Verification items for the finished model (mm, model axes). Face numbers are marked on the shaded views. A direction names the side the tool comes from. Coordinates: 2 decimals unless noted, no trailing zeros. Write each loop counter-clockwise with the first axis right and the second up, starting at its lowest first coordinate (ties: lowest second). Pieces come first, ordered by that corner, then holes. Notation, with made-up numbers: (6, 47) - (51, 47) arc R11 ccw to (51, 56) - close; hole circle Ø11 at (22, 68.5). An arc over 180 degrees is marked (long way). Use CSV: the item, a comma, the result in double quotes. Start each with the question number.
```python
from build123d import *

# Parameters (mm, degrees)
F0_R     = 9.5
F1_DEPTH = 20
F2_DEPTH = 15


with BuildPart() as f1:
    # F0 (on Top) → F1 (new body)
    with BuildSketch(Plane.XY):
        with BuildLine():
            ThreePointArc((11, 0), (2.57123, 10.695269), (-9.797959, 5))
            ThreePointArc((-9.797959, 5), (-11, 0), (-9.797959, -5))
            ThreePointArc((-9.797959, -5), (2.57123, -10.695269), (11, 0))
        make_face()
        Circle(F0_R, mode=Mode.SUBTRACT)
    extrude(amount=F1_DEPTH)

    # F0 (on Top) → F2 (join)
    with BuildSketch(Plane.XY):
        with BuildLine():
            Line((-9.797959, 5), (-24.797959, 5))
            Line((-24.797959, 5), (-24.797959, -5))
            Line((-24.797959, -5), (-9.797959, -5))
            ThreePointArc((-9.797959, -5), (-11, 0), (-9.797959, 5))
        make_face()
    extrude(amount=F2_DEPTH)


solid = f1.part
```
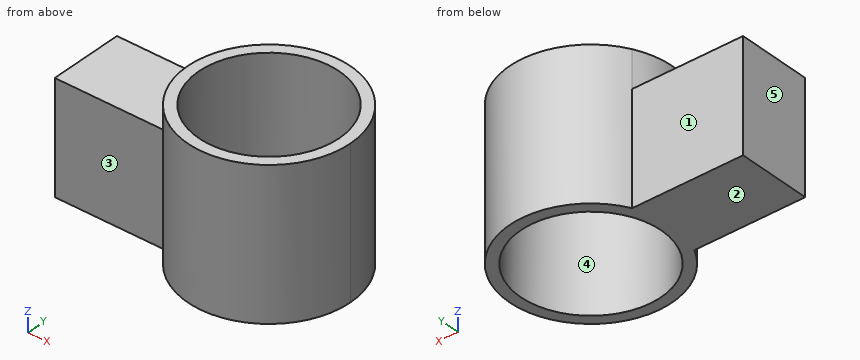
Q1. Cross-section at D-D (x = -8.5). Record the cut outline in (y, z), plus the area to 3 significant figures.
Q2. Gauge pin test, flat ends, axial feed: pin 1 (1 mm diameter, centred on x = 3, z = 11, fed in from -Y); pin 2 (10 mm diameter, centred on x = 2.5, z = 14.5, fed in from -Y); pin 3 (1 mm diameter, centred on y = 6.5, z = 6, fed in from -X); pin 4 (1 mm diameter, centred on x = -16.5, z = 9, fed in from +Y). Record the tip position at first contact, or that the pin passes through.
Q3. Release check for a two-part mould opening along X. For the marked faces 3, 4 and 5 record: released by +X, released by -X, zero draft, split by the parting line, or undercut.
Q4. Cross-section at A-A (x = 0). Record the cut outline in (y, z).
Q5. Tool access check on the marked faces 1 and 2. Record the directions out of +Z, -Z, +X, -X, +Y, -Y that give a thin tool (end or side, any length) a straight path to the whole face; none if there is none.
Q6. Scan lines: line 1 along Y through (x, z) = (0, 5.25); line 2 along Y through (x, z) = (-12, 12.25); line 3 along Y through (x, z) = (3, 8.75). Record each from-to range of solid material in increasing order. Write a range as from..to.
Q7. Cross-section at C-C (y = -4.5). Record the cut outline in (x, z).
Q8. Cross-section at B-B (z = 8.75). Record the cut outline in (x, y), plus the area to 3 significant figures.
Reply:
1,outline,"(-6.98, 0) - (-4.24, 0) - (-4.24, 20) - (-6.98, 20) - close; (4.24, 0) - (6.98, 0) - (6.98, 20) - (4.24, 20) - close"
1,area,"110 mm^2"
2,pin 1,"y = -10.71"
2,pin 2,"y = -11"
2,pin 3,"x = -9.22"
2,pin 4,"y = 5"
3,face 3,"zero draft"
3,face 4,"undercut"
3,face 5,"released by -X"
4,outline,"(-11, 0) - (-9.5, 0) - (-9.5, 20) - (-11, 20) - close; (9.5, 0) - (11, 0) - (11, 20) - (9.5, 20) - close"
5,face 1,"+Z, -Z, -X, +Y"
5,face 2,"-Z, +X, -X, +Y, -Y"
6,line 1,"-11..-9.5, 9.5..11"
6,line 2,"-5..5"
6,line 3,"-10.58..-9.01, 9.01..10.58"
7,outline,"(-24.8, 0) - (-8.37, 0) - (-8.37, 20) - (-10.04, 20) - (-10.04, 15) - (-24.8, 15) - close; (8.37, 0) - (10.04, 0) - (10.04, 20) - (8.37, 20) - close"
8,outline,"(-24.8, -5) - (-9.8, -5) arc R11 ccw (long way) to (-9.8, 5) - (-24.8, 5) - close; hole circle Ø19 at (0, 0)"
8,area,"238 mm^2"
